Could you check a few things on this model? Use its own coordinates, in mm. Face numbers are marked on the shaded views. A direction names the side the tool comes from. Give positions to 0.01 mm unless a question says otherwise; leave off trailing zeros. Write each loop counter-clockwise with the first axis right and the second up, starting at its lowest first coordinate (ties: lowest second). Pieces come first, ordered by that corner, then holes. Notation, with made-up numbers: (31, 49) - (51, 49) arc R21 cw to (51, 74) - close; hole circle Ø9 at (83, 82). An arc over 180 degrees is marked (long way). Write item = value, one per line.
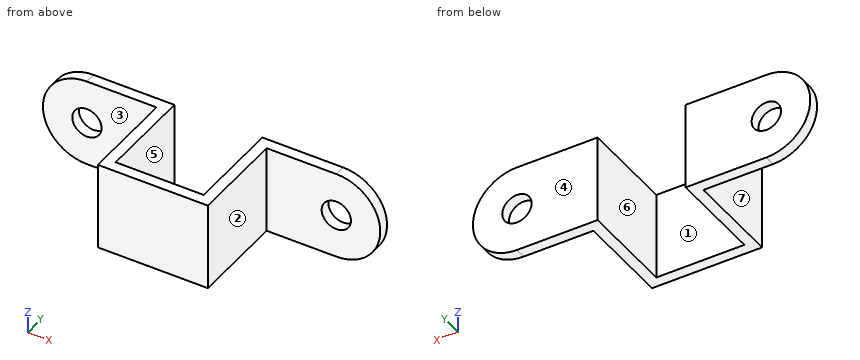
from build123d import *

# Parameters (mm, degrees)
F1_DEPTH      = 19.05
F1_DEPTH_BACK = 19.05
F3_D          = 12.7
F2_R          = 19.05
F2_R_2        = 6.35
F4_DEPTH      = 4.7625


with BuildPart() as f1:
    # F0 (on Top) → F1 (new body, two sides)
    with BuildSketch(Plane.XY) as f1_sk:
        Polygon((-19.05, -41.275), (-19.05, 0), (-53.975, 0), (-53.975, -4.7625), (-23.8125, -4.7625), (-23.8125, -46.0375), (23.8125, -46.0375), (23.8125, -4.7625), (53.975, -4.7625), (53.975, 0), (19.05, 0), (19.05, -41.275), align=None)
    extrude(amount=F1_DEPTH)
    extrude(f1_sk.sketch, amount=-F1_DEPTH_BACK)

    # F3 (through all)
    with Locations(Plane(origin=(0, 0, 0), x_dir=(1, 0, 0), z_dir=(0, 1, 0))):
        with Locations((-53.975, 0), (53.975, 0)):
            Hole(F3_D / 2)

    # F2 (on Front) → F4 (join)
    with BuildSketch(Plane.XZ):
        with Locations((-53.975, 0)):
            Circle(F2_R)
        with Locations((-53.975, 0)):
            Circle(F2_R_2, mode=Mode.SUBTRACT)
        with Locations((53.975, 0)):
            Circle(F2_R)
        with Locations((53.975, 0)):
            Circle(F2_R_2, mode=Mode.SUBTRACT)
    extrude(amount=F4_DEPTH)


solid = f1.part
1. I need wall thicknesses on line 1 (X direction, y = -38.5, z = -11); line 2 (Y direction, x = 44, z = 9); line 3 (Y direction, x = -12, z = -10) (1 decimal). Which ranges of each line are inside material? Lowest first, please.
Filled sheet:
line_1 = -23.81 to -19.05, 19.05 to 23.81
line_2 = -4.76 to 0
line_3 = -46 to -41.3
2. If we section it at B-B, the plane z = 0: Count the separate pieces of the cut face and the enclosed holes in it, and give its area (3 significant figures).
Filled sheet:
separate_pieces = 3
enclosed_holes = 0
area = 968 mm2
3. Thinking about a two-plate mould opening in X: for the marked faces 4, 5, 6 and 7, which applies, pulls with the +X half, pulls with the -X half, needs draft (parallel to the pull), parting line crosses it, or undercut?
Filled sheet:
face_4 = needs draft
face_5 = undercut
face_6 = undercut
face_7 = pulls with the -X half
4. If we section it at A-A, the plane y = -22: Please give me the cut outline in (x, z), and give its area (3 significant figures).
Filled sheet:
outline = (-23.81, -19.05) - (-19.05, -19.05) - (-19.05, 19.05) - (-23.81, 19.05) - close; (19.05, -19.05) - (23.81, -19.05) - (23.81, 19.05) - (19.05, 19.05) - close
area = 363 mm2
5. If we section it at C-C, the plane x = 56.5: Please give me the cut outline in (y, z).
Filled sheet:
outline = (-4.76, -18.88) - (0, -18.88) - (0, -5.83) - (-4.76, -5.83) - close; (-4.76, 5.83) - (0, 5.83) - (0, 18.88) - (-4.76, 18.88) - close
6. Which directions (+Z, -Z, +X, -X, +Y, -Y) give clear straight access to the entire face, cutting with the end or side of a thin tool? Please do the marked faces 1, 2 and 3.
Filled sheet:
face_1 = +Z, -Z, +Y
face_2 = +Z, -Z, +X, -Y
face_3 = +Z, -Z, -X, -Y
7. For pin 1 (3 mm diameter, centred on y = -31, z = 14.5, fed in from +X); pin 2 (2 mm diameter, centred on x = 17, z = 3, fed in from +Y) (3 decimals); pin 3 (19 mm diameter, centred on x = 44, z = -1.5, fed in from -Y), each with a flat end and sliding along its axis, tell me the tip position at first contact or that it passes through.
Filled sheet:
pin_1 = 23.81
pin_2 = -41.275
pin_3 = -4.76
